Read the model definition and answer for the solid it produces. Units are mm, in the model's axes. Face numbers are marked on the shaded views. Coordinates: 2 decimals unless noted, no trailing zeros. Write each loop counter-clockwise with the first axis right and the second up, starting at its lowest first coordinate (ties: lowest second). Pieces come first, ordered by that corner, then holes. Notation, with made-up numbers: (-30, 58) -> (-4, 58) arc R22 ccw to (-4, 65) -> close; hole circle Ø6 at (23, 84). An arc over 180 degrees is marked (long way). Answer in a Markdown table with one row per item. Add a question column.
Item 1: Section D-D on y = 70 is taken. Write down the section's boundary in (x, z), then the cut area to 3 significant figures.
Item 2: Straight lines are drawn through the part: line 1 (Y direction, x = -6, z = 2); line 2 (Y direction, x = -2.5, z = 5.75); line 3 (Z direction, x = -6, y = 37). For each, find the intervals that lie inside material, in ascending order. Write a range as from..to.
Item 3: Section B-B on y = -75 is taken. Write down the section's boundary in (x, z).
Item 4: For a pull along Y with two mould halves and no side action, classify the marked faces 1 and 2 as +Y half, -Y half, draft (parallel to the pull), parting line (faces both ways), or undercut.
Item 5: Section A-A on z = 6.25 is taken. Write down the section's boundary in (x, y), then the cut area to 3 significant figures.
Item 6: Given pin 1 Ø2.5 at (x, y) = (-4, -74) entering from +Z; pin 2 Ø6 at (x, y) = (-2.5, -22) entering from +Z; pin 3 Ø7.5 at (y, z) = (34, 10.5) entering from -X, each flat-ended and moving along its own axis, determine where each tip first touches the part or whether it passes through.
Item 7: Section C-C on x = -9.25 is taken. Write down the section's boundary in (y, z), then the cut area to 3 significant figures.
```python
from build123d import *

# Parameters (mm, degrees)
SKETCH_1_W                       = 25
SKETCH_1_H                       = 210
SM_BASE_FLANGE_1_DEPTH           = 3
SM_EDGE_FLANGE_1_STRIP_W         = 16
SM_EDGE_FLANGE_1_STRIP_H         = 3
SM_EDGE_FLANGE_1_STRIP_CUT_DEPTH = 210
SM_EDGE_FLANGE_1_DEPTH           = 210
SKETCH_9_R                       = 2.5
EXTRUDE_1_DEPTH                  = 15
FILLET_1_R                       = 5


# Sheet-metal steps are written as plain solids
with BuildPart() as part:
    # Sketch 1 → 基体-法兰1 (new body)
    with BuildSketch(Plane.XY):
        Rectangle(SKETCH_1_W, SKETCH_1_H)
    extrude(amount=-SM_BASE_FLANGE_1_DEPTH)

    # 边线-法兰1 strip (across the edge) → 边线-法兰1 strip cut (cut)
    with BuildSketch(Plane(origin=(12.5, -105, 0), x_dir=(-1, 0, 0), z_dir=(0, 1, 0))):
        with Locations((-3, -1.5)):
            Rectangle(SM_EDGE_FLANGE_1_STRIP_W, SM_EDGE_FLANGE_1_STRIP_H)
    extrude(amount=SM_EDGE_FLANGE_1_STRIP_CUT_DEPTH, mode=Mode.SUBTRACT)

    # 边线-法兰1 section (across the edge) → 边线-法兰1 (add)
    with BuildSketch(Plane(origin=(12.5, -105, 0), x_dir=(-1, 0, 0), z_dir=(0, 1, 0))):
        with BuildLine():
            Line((0, 2), (0, 17))
            Line((0, 17), (3, 17))
            Line((3, 17), (3, 2))
            ThreePointArc((3, 2), (3.585786438, 0.585786438), (5, 0))
            Line((5, 0), (5, -3))
            ThreePointArc((5, -3), (1.464466094, -1.535533906), (0, 2))
        make_face()
    extrude(amount=SM_EDGE_FLANGE_1_DEPTH)

    # 草图9 → 凸台-拉伸1 (add)
    with BuildSketch(Plane.XY):
        with Locations((-4.5, 0)):
            Circle(SKETCH_9_R)
        with Locations((-4.5, -75)):
            Circle(SKETCH_9_R)
        with Locations((-4.5, 75)):
            Circle(SKETCH_9_R)
    extrude(amount=EXTRUDE_1_DEPTH)

    # 圆角1
    fillet_1_edges = [part.edges().sort_by_distance(p)[0] for p in [
        (11, -105, 17),
        (11, 105, 17),
        (-12.5, -105, -1.5),
        (-12.5, 105, -1.5),
    ]]
    fillet(fillet_1_edges, radius=FILLET_1_R)


solid = part.part
```
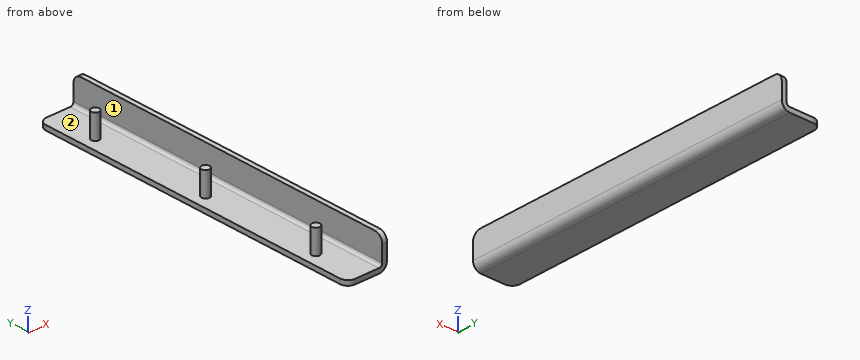
Results below:
| question | item | result |
|---|---|---|
| 1 | outline | (-12.5, -3) -> (7.5, -3) arc R5 ccw to (12.5, 2) -> (12.5, 17) -> (9.5, 17) -> (9.5, 2) arc R2 cw to (7.5, 0) -> (-12.5, 0) -> close |
| 1 | area | 121 mm2 |
| 2 | line 1 | y = -77..-73, -2..2, 73..77 |
| 2 | line 2 | y = -76.5..-73.5, -1.5..1.5, 73.5..76.5 |
| 2 | line 3 | z = -3..0 |
| 3 | outline | (-12.5, -3) -> (7.5, -3) arc R5 ccw to (12.5, 2) -> (12.5, 17) -> (9.5, 17) -> (9.5, 2) arc R2 cw to (7.5, 0) -> (-2, 0) -> (-2, 15) -> (-7, 15) -> (-7, 0) -> (-12.5, 0) -> close |
| 4 | face 1 | draft |
| 4 | face 2 | undercut |
| 5 | outline | circle Ø5 at (-4.5, -75); circle Ø5 at (-4.5, 0); circle Ø5 at (-4.5, 75); (9.5, -105) -> (12.5, -105) -> (12.5, 105) -> (9.5, 105) -> close |
| 5 | area | 689 mm2 |
| 6 | pin 1 | stops at z = 15 |
| 6 | pin 2 | stops at z = 0 |
| 6 | pin 3 | stops at x = 9.5 |
| 7 | outline | (-104.68, -3) -> (104.68, -3) -> (104.68, 0) -> (-104.68, 0) -> close |
| 7 | area | 628 mm2 |
